Here's how the part is built. I have some questions about the finished solid (model axes, mm). A direction names the side the tool comes from. Round coordinates to 2 decimals unless told otherwise and drop trailing zeros. Order: outer loops, then holes, each group sorted by start corner. A loop starts at its lowest first (then second) coordinate and runs counter-clockwise, first axis right, second up.
```python
from build123d import *

# Parameters (mm, degrees)
SKETCH_W     = 10
SKETCH_H     = 10
PAD_DEPTH    = 5
SKETCH001_R  = 10.375
PAD001_DEPTH = 6


with BuildPart() as part:
    # Sketch → Pad (new body)
    with BuildSketch(Plane.XY.offset(6)):
        Rectangle(SKETCH_W, SKETCH_H)
    extrude(amount=PAD_DEPTH)

    # Sketch001 → Pad001 (join)
    with BuildSketch(Plane.XY):
        Circle(SKETCH001_R)
    extrude(amount=PAD001_DEPTH)


solid = part.part
```
1) For faces 1 (the flat face through (0, 0, 11)), 2 (the flat face through (-5, 0, 8)), 3 (the flat face through (0, 5, 8)), 4 (the flat face through (0, -5, 8)), 5 (the flat face through (5, 0, 8)), which set-ups out of +Z, -Z, +X, -X, +Y, -Y let a thin tool reach every point of the face, with its end or its side?
2) I need wall thicknesses on line 1 (X direction, y = 3, z = 10.75); line 2 (Z direction, x = -5.75, y = -7.5). Which ranges of each line are inside material? Lowest first, please.
3) I'm going to push flat-ended pins straight in: pin 1 (1.5 mm diameter, centred on y = 0, z = 7.5, fed in from +X); pin 2 (2.5 mm diameter, centred on y = -2, z = 9.5, fed in from -X); pin 3 (4 mm diameter, centred on y = 4, z = 7, fed in from -X); pin 4 (1.5 mm diameter, centred on y = 6.5, z = 7.5, fed in from +X). Where does each tip first touch, or does it pass through?
4) If we section it at A-A (y = 0): Write out the boundary of the cut face in (x, z) (3 decimals).
5) If we section it at C-C (z = 10.25): Write out the boundary of the cut face in (x, y), plus the area to 3 significant figures.
6) If we section it at D-D (z = 1): Write out the boundary of the cut face in (x, y) (3 decimals), plus the area to 3 significant figures.
Solutions:
1. face 1: +Z, +X, -X, +Y, -Y
1. face 2: +Z, -X, +Y, -Y
1. face 3: +Z, +X, -X, +Y
1. face 4: +Z, +X, -X, -Y
1. face 5: +Z, +X, +Y, -Y
2. line 1: x = -5 to 5
2. line 2: z = 0 to 6
3. pin 1: stops at x = 5
3. pin 2: stops at x = -5
3. pin 3: stops at x = -10.12
3. pin 4: passes through
4. outline: (-10.375, 0) - (10.375, 0) - (10.375, 6) - (5, 6) - (5, 11) - (-5, 11) - (-5, 6) - (-10.375, 6) - close
5. outline: (-5, -5) - (5, -5) - (5, 5) - (-5, 5) - close
5. area: 100 mm2
6. outline: circle Ø20.75 at (0, 0)
6. area: 338 mm2
